from build123d import *

# Parameters (mm, degrees)
SKETCH1_W           = 233.68
SKETCH1_H           = 101.6
BOSS_EXTRUDE1_DEPTH = 508
CUT_EXTRUDE1_DEPTH  = 569.324645251
CUT_EXTRUDE2_DEPTH  = 569.324645251
CUT_EXTRUDE3_DEPTH  = 569.324645251
CUT_EXTRUDE4_DEPTH  = 538.880617648


with BuildPart() as part:
    # Sketch1 → Boss-Extrude1 (new body)
    with BuildSketch(Plane.XY):
        with Locations((-116.84, 50.8)):
            Rectangle(SKETCH1_W, SKETCH1_H)
    extrude(amount=-BOSS_EXTRUDE1_DEPTH)

    # Sketch2 → Cut-Extrude1 (cut, through all)
    with BuildSketch(Plane.XY):
        Polygon((-202.283526953, 101.6), (-233.68, 73.908067848), (-233.68, 101.6), align=None)
        Polygon((-202.283526953, 0), (-233.68, 26.611014762), (-233.68, 0), align=None)
    extrude(amount=-CUT_EXTRUDE1_DEPTH, mode=Mode.SUBTRACT)

    # Sketch3 → Cut-Extrude2 (cut, through all)
    with BuildSketch(Plane(origin=(0, 101.6, 0), x_dir=(1, 0, 0), z_dir=(0, 1, 0))):
        Polygon((-87.070770682, 508), (-233.68, 321.585732495), (-233.68, 508), align=None)
    extrude(amount=-CUT_EXTRUDE2_DEPTH, mode=Mode.SUBTRACT)

    # Sketch4 → Cut-Extrude3 (cut, through all)
    with BuildSketch(Plane(origin=(0, 0, 0), x_dir=(0, 0, -1), z_dir=(1, 0, 0))):
        Polygon((463.161638797, 101.6), (508, 80.157516446), (508, 101.6), align=None)
        Polygon((463.161638797, 0), (508, 21.319923331), (508, 0), align=None)
    extrude(amount=-CUT_EXTRUDE3_DEPTH, mode=Mode.SUBTRACT)

    # Sketch5 → Cut-Extrude4 (cut, through all)
    with BuildSketch(Plane(origin=(217.205760792, 0, -275.127297003), x_dir=(-0.7848827655334263, 1.8564028129682992e-15, -0.6196442885790207), z_dir=(0.6196442885790207, 2.3514435630931796e-15, -0.7848827655334263))):
        Polygon((351.862738174, 101.6), (383.119645888, 76.175565291), (383.013937726, 101.6), align=None)
        Polygon((383.119645888, 27.634188335), (351.862738174, 0), (383.013937726, 0), align=None)
    extrude(amount=-CUT_EXTRUDE4_DEPTH, mode=Mode.SUBTRACT)


with BuildPart() as cut_extrude4_kept_piece:
    # of the separate pieces the step leaves, the one the design keeps (cut_extrude4_pieces_kept)
    add(part.part.solids().sort_by_distance((0, 0, 0))[0])


solid = cut_extrude4_kept_piece.part
Here's how the part is built. I have some questions about the finished solid (model axes, mm). Coordinates: 2 decimals unless noted, no trailing zeros. Write each loop counter-clockwise with the first axis right and the second up, starting at its lowest first coordinate (ties: lowest second). Pieces come first, ordered by that corner, then holes.
1) If we section it at C-C (z = -247.5): List the corners of the cut face in (x, y) for me, plus the area to 3 significant figures.
Filled in:
outline: (-233.68, 26.61) - (-202.28, 0) - (0, 0) - (0, 101.6) - (-202.28, 101.6) - (-233.68, 73.91) - close
area: 22,900 mm2
2) If I drill on line 1 (X direction, y = 19, z = -410); line 2 (Y direction, x = -220, z = -110.5); line 3 (X direction, y = 48, z = -402.5), over which ranges is the centre line in solid material (lowest first)?
Filled in:
line 1: x = -152 to 0
line 2: y = 15.02 to 85.97
line 3: x = -170.04 to 0
3) If we section it at D-D (y = 87.5): List the corners of the cut face in (x, z) for me.
Filled in:
outline: (-218.27, -319.35) - (-81.45, -492.65) - (0, -492.65) - (0, 0) - (-218.27, 0) - close
4) If we section it at A-A (x = -70): List the corners of the cut face in (y, z) for me, plus the area to 3 significant figures.
Filled in:
outline: (0, -463.16) - (21.32, -508) - (80.16, -508) - (101.6, -463.16) - (101.6, 0) - (0, 0) - close
area: 50,700 mm2
5) If we section it at B-B (y = 33): List the corners of the cut face in (x, z) for me.
Filled in:
outline: (-233.68, -321.59) - (-87.07, -508) - (0, -508) - (0, 0) - (-233.68, 0) - close
6) I'm going to push flat-ended pins straight in: pin 1 (5 mm diameter, centred on x = -65, y = 17, fed in from -Z); pin 2 (2 mm diameter, centred on x = -94, y = 53, fed in from -Z). Where does each tip first touch, or does it pass through?
Filled in:
pin 1: stops at z = -504.17
pin 2: stops at z = -500.46
